Could you check a few things on this drawing? It's one solid part, dimensions in mm from its lowest x, y, z. A direction names the side the tool comes from. Give positions to 0.01 mm unless a question says otherwise; leave off trailing zeros. Loops run counter-clockwise (first coordinate to the right, second up) from the corner with the lowest first, then second, coordinate; pieces in that order, holes last. Notation, with made-up numbers: (9, 33.25) - (29, 33.25) arc R7 ccw to (29, 45.25) - close; hole circle Ø11 at (84, 84). An arc over 180 degrees is marked (long way). Return JSON: item names as keys, results as strings. Group by question number.
(1) If we section it at C-C (z = 67): Please give me the cut outline in (x, y) (1 decimal).
(2) If we section it at A-A (z = 30): Please give me the cut outline in (x, y) (1 decimal), then the cut area to 3 significant figures.
(3) On a 3-axis mill with a long thin cutter (end or side, diameter ignored), from which of +Z, -Z, +X, -X, +Y, -Y can I reach the whole of each face in a straight line? I mean the marked faces 1 and 2. Say none if no direction works.
(4) For P1, Ø2, axis at x = 55.5, z = 47.5, coming from the -Y side; P2, Ø0.8, axis at y = 4, z = 19, coming from the +X side (3 decimals); P3, Ø2, axis at y = 0.5, z = 35, coming from the -X side; P4, Ø1.3, axis at x = 89.5, y = 1.5, coming from the +Z side, each with a flat end and sliding along its axis, tell me the tip position at first contact or that it passes through.
(5) If we section it at B-B (x = 6): Please give me the cut outline in (y, z).
(6) I need wall thicknesses on probe 1 along Y at (x, z) = (43.5, 64); probe 2 along X at (y, z) = (3.2, 26) (1 decimal); probe 3 along X at (y, z) = (1.1, 42) (1 decimal). Which ranges of each line are inside material? Lowest first, please. Write a range as [from, to].
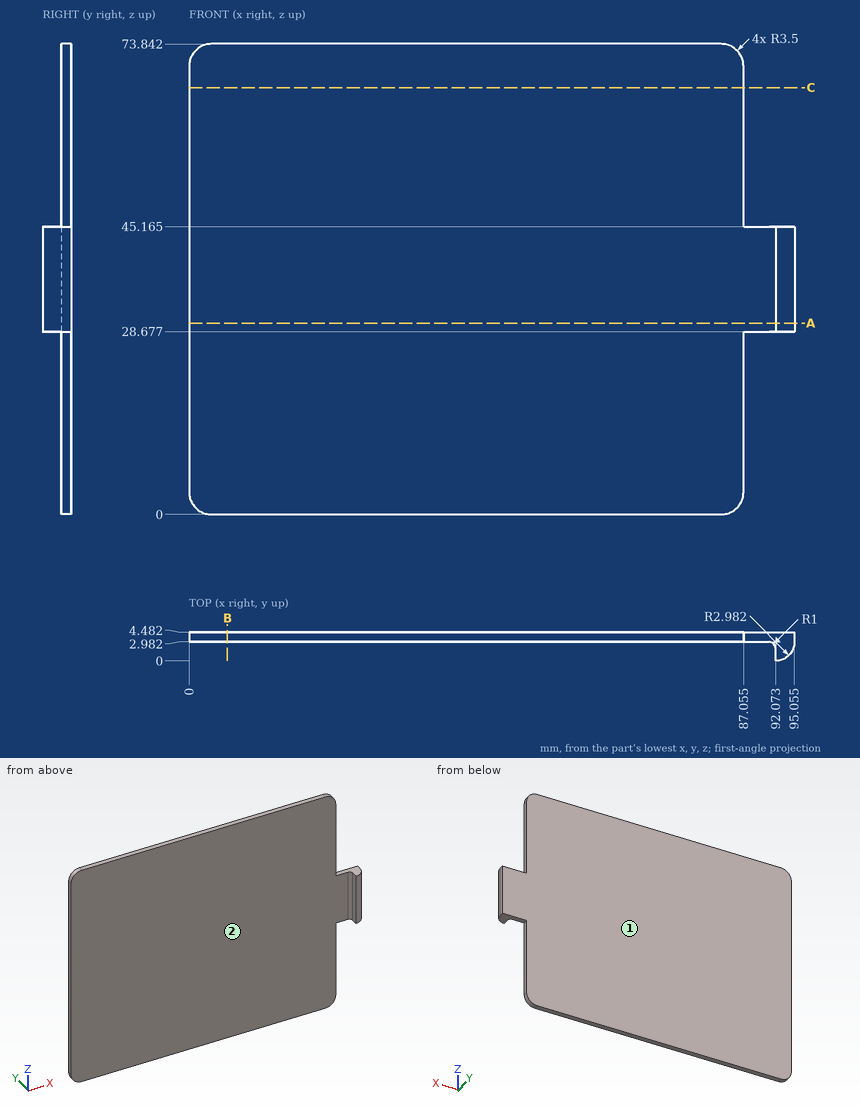
Values:
{
 "1": {"outline": "(0, 3) - (87.1, 3) - (87.1, 4.5) - (0, 4.5) - close"},
 "2": {"outline": "(0, 3) - (91.1, 3) arc R1 cw to (92.1, 2) - (92.1, 0) arc R3 ccw to (95.1, 3) - (95.1, 4.5) - (0, 4.5) - close", "area": "150 mm2"},
 "3": {"face 1": "+Z, -Z, +X, -X, +Y", "face 2": "+Z, -Z, -X, -Y"},
 "4": {"P1": "y = 2.98", "P2": "x = 87.055", "P3": "x = 92.07", "P4": "through"},
 "5": {"outline": "(2.98, 0) - (4.48, 0) - (4.48, 73.84) - (2.98, 73.84) - close"},
 "6": {"probe 1": "[2.98, 4.48]", "probe 2": "[0, 87.1]", "probe 3": "[92.1, 94.4]"}
}
